Solid Edge part; units mm, degrees
sketch "Sketch1" plane through (0, 0, 0) normal (0, -1, 0) x (1, 0, 0)
  line L0 (37.5, 0) -> (0, 0)
  line L1 (0, 0) -> (0, 15)
  line L2 (0, 15) -> (37.5, 15)
  line L3 (37.5, 15) -> (37.5, 0)
extrude "Protrusion1" add sketch "Sketch1" along normal blind 5
sketch "Sketch2" plane through (18.75, 0, 7.5) normal (0, 1, 0) x (-1, 0, 0)
  line L0 (13.75, -7.5) -> (13.75, 7.5)
  line L1 (13.75, 7.5) -> (18.75, 7.5)
  line L2 (18.75, 7.5) -> (18.75, -7.5)
  line L3 (18.75, -7.5) -> (13.75, -7.5)
extrude "ExtrudedProtrusion_3" add sketch "Sketch2" along normal blind 15
sketch "Sketch3" plane through (0, 5, 7.5) normal (-1, 0, 0) x (0, -1, 0)
  circle A0 centre (-3, 0) radius 4
extrude "Cutout1" cut sketch "Sketch3" against normal through all
fillet "Round1" radius 7 2 edges at (2.5, 15, 15) (2.5, 15, 0)
mirror "Mirror1" about plane through (18.75, 5, 7.5) normal (-1, 0, 0) of "ExtrudedProtrusion_3", "Cutout1"
fillet "Round2" radius 7 2 edges at (35, 15, 15) (35, 15, 0)
Source: CAD feature listing. Evaluate the final solid. Frame: model axes, mm. A direction names the side the tool comes from. Give positions to 0.01 mm unless a question says otherwise; leave off trailing zeros. Order: outer loops, then holes, each group sorted by start corner. A loop starts at its lowest first (then second) coordinate and runs counter-clockwise, first axis right, second up. Notation, with made-up numbers: (81.5, 21.5) -> (137.5, 21.5) arc R22 ccw to (137.5, 35.5) -> close; hole circle Ø3 at (-8, -33). An arc over 180 degrees is marked (long way). Write item = value, one per line.
Item 1: Section query A-A (y = 2). Output: boundary loops of the cut face in (x, z).
Check result:
outline = (0, 0) -> (5, 0) -> (5, 15) -> (0, 15) -> close; (32.5, 0) -> (37.5, 0) -> (37.5, 15) -> (32.5, 15) -> close
Item 2: Set-up query: faces 5 (the face through (32.5, 4, 9)), 6 (the face through (2.5, 12.9, 13)). Return all of +Z, -Z, +X, -X, +Y, -Y with unobstructed straight access to the full face (end or side cutting, diameter ignored); none if empty.
Check result:
face_5 = +Z, -Z, +Y
face_6 = +Z, +X, -X, +Y
Item 3: Ray query, probe 1 along Z at (x, y) = (34.5, 8); probe 2 along Y at (x, z) = (35.25, 7.5); probe 3 along X at (y, z) = (1, 4). Return the intervals inside material, ascending.
Check result:
probe_1 = 0 to 3.5, 11.5 to 15
probe_2 = -5 to 4, 12 to 15
probe_3 = 0 to 5, 32.5 to 37.5
Item 4: Mould query, pull axis Z, two halves, no side actions, for faces 1 (the face through (18, -1, 15)), 2 (the face through (2.5, 15, 7.5)), 3 (the face through (2.5, 11.2, 5.1)), 4 (the face through (35.035, 11.996, 7.324)). Classes: +Z half, -Z half, draft (parallel to the pull), parting line (faces both ways), or undercut.
Check result:
face_1 = +Z half
face_2 = draft
face_3 = undercut
face_4 = undercut
Item 5: Section query D-D (y = 9.25). Output: boundary loops of the cut face in (x, z).
Check result:
outline = (0, 0.11) -> (5, 0.11) -> (5, 3.7) -> (0, 3.7) -> close; (0, 11.3) -> (5, 11.3) -> (5, 14.89) -> (0, 14.89) -> close; (32.5, 0.11) -> (37.5, 0.11) -> (37.5, 3.7) -> (32.5, 3.7) -> close; (32.5, 11.3) -> (37.5, 11.3) -> (37.5, 14.89) -> (32.5, 14.89) -> close
Item 6: Contact query for flat-ended pins moving along their axis: pin 1 (6 mm diameter, centred on x = 18.5, z = 11.5, fed in from +Y); pin 2 (8 mm diameter, centred on x = 23.5, y = 5.5, fed in from +Z) (3 decimals). Output: stop coordinate, or through.
Check result:
pin_1 = 0
pin_2 = through
Item 7: Section query B-B (x = 34.5). Output: boundary loops of the cut face in (y, z), then the cut area to 3 significant figures.
Check result:
outline = (-5, 0) -> (8, 0) arc R7 ccw to (15, 7) -> (15, 8) arc R7 ccw to (8, 15) -> (-5, 15) -> close; hole circle Ø8 at (8, 7.5)
area = 229 mm²
Item 8: Section query C-C (z = 12.25). Output: boundary loops of the cut face in (x, y), then the cut area to 3 significant figures.
Check result:
outline = (0, -5) -> (37.5, -5) -> (37.5, 13.56) -> (32.5, 13.56) -> (32.5, 0) -> (5, 0) -> (5, 13.56) -> (0, 13.56) -> close
area = 323 mm²
